Part model, mm, in its own coordinate system. Face numbers are marked on the shaded views. A direction names the side the tool comes from. Coordinates: 2 decimals unless noted, no trailing zeros. Loops run counter-clockwise (first coordinate to the right, second up) from the corner with the lowest first, then second, coordinate; pieces in that order, holes last. Notation, with made-up numbers: M 31,-8.5 L 72,-8.5 A20 cw 72,1.5 Z; hole C 7.5,58.5 d5. An arc over 180 degrees is marked long. Use a Markdown table: item, result. Add a question column.
1) Band-saw the part on C-C (z = -102.5). List the corners of the cut face in (x, y).
2) Tool access for the marked faces 1 and 2: list every direction of +Z, -Z, +X, -X, +Y, -Y with a clear straight run to the whole face (end or side of a thin tool).
3) Pin check, flat tips, straight feed: pin 1 Ø6 at (y, z) = (-45, -134.5) entering from +X; pin 2 Ø4 at (y, z) = (-28, -86) entering from -X; pin 3 Ø6 at (y, z) = (-46.5, -132.5) entering from -X. Stop position of each tip, or through.
4) Band-saw the part on B-B (y = 11). List the corners of the cut face in (x, z).
5) Band-saw the part on A-A (x = 0). List the corners of the cut face in (y, z).
6) Band-saw the part on D-D (y = -19). List the corners of the cut face in (x, z), plus the area to 3 significant figures.
7) Wall check: probe 1 along Y at (x, z) = (0, -138.5); probe 2 along X at (y, z) = (0, -142); probe 3 along Y at (x, z) = (0, -81). Give the ranges that are in metal, low to high. Write a range as from..to.
from build123d import *

# Parameters (mm, degrees)
SHELL1_T           = 3
SKETCH5_R          = 25
CUT_EXTRUDE3_DEPTH = 170.883652636
SKETCH6_W          = 64
SKETCH6_H          = 41
CUT_EXTRUDE4_DEPTH = 170.883652636


with BuildPart() as part:
    # Sketch2 → Revolve1 (revolve)
    with BuildSketch(Plane(origin=(0, 0, 0), x_dir=(0, 0, -1), z_dir=(1, 0, 0)), mode=Mode.PRIVATE) as revolve1_sk:
        with BuildLine():
            Line((76.080335522, 0), (147.580335522, 0))
            Line((147.580335522, 0), (147.580335522, 56.5))
            Line((147.580335522, 56.5), (132.580335522, 56.5))
            ThreePointArc((132.580335522, 56.5), (92.628802385, 39.951533137), (76.080335522, 0))
        make_face()
    revolve(revolve1_sk.sketch.rotate(Axis((0, 0, -76.080335522), (0, 0, 1)), 90), axis=Axis((0, 0, -76.080335522), (0, 0, 1)))

    # Shell1
    shell1_openings = [part.faces().sort_by_distance(p)[0] for p in [
        (0, 0, -147.580335522),
    ]]
    offset(amount=SHELL1_T, openings=shell1_openings, kind=Kind.INTERSECTION)

    # Sketch5 → Cut-Extrude3 (cut, through all)
    with BuildSketch(Plane.XY):
        with Locations(Location((0, 0, 0), (0, 0, 180))):
            Circle(SKETCH5_R)
    extrude(amount=-CUT_EXTRUDE3_DEPTH, mode=Mode.SUBTRACT)

    # Sketch6 → Cut-Extrude4 (cut, through all)
    with BuildSketch(Plane(origin=(0, 0, 0), x_dir=(1, 0, 0), z_dir=(0, 1, 0))):
        with Locations((0, 127.080335522)):
            Rectangle(SKETCH6_W, SKETCH6_H)
    extrude(amount=-CUT_EXTRUDE4_DEPTH, mode=Mode.SUBTRACT)


solid = part.part
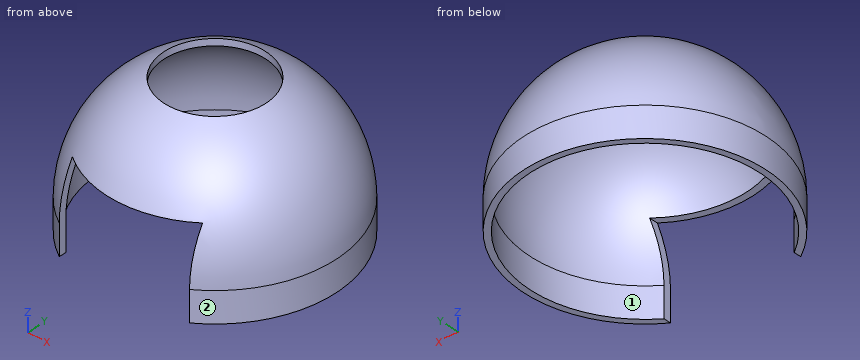
Entries:
| question | item | result |
|---|---|---|
| 1 | outline | C 0,0 d102.67; hole C 0,0 d95.65 |
| 2 | face 1 | -Z |
| 2 | face 2 | +Z, -Z |
| 3 | pin 1 | x = 42.15 |
| 3 | pin 2 | x = -28.28 |
| 3 | pin 3 | x = -40.6 |
| 4 | outline | M -58.47,-147.58 L -55.42,-147.58 L -55.42,-132.58 A55.42 cw -22.45,-81.91 L -22.45,-78.59 A58.47 ccw -58.47,-132.58 Z; M 22.45,-81.91 A55.42 cw 55.42,-132.58 L 55.42,-147.58 L 58.47,-147.58 L 58.47,-132.58 A58.47 ccw 22.45,-78.59 Z |
| 5 | outline | M -53.52,-106.58 L -50.16,-106.58 A56.5 cw -25,-81.91 L -25,-78.59 A59.5 ccw Z; M 25,-81.91 A56.5 cw 56.5,-132.58 L 56.5,-147.58 L 59.5,-147.58 L 59.5,-132.58 A59.5 ccw 25,-78.59 Z |
| 6 | outline | M -56.38,-147.58 L -53.21,-147.58 L -53.21,-132.58 A53.21 cw -16.25,-81.91 L -16.25,-78.59 A56.38 ccw -56.38,-132.58 Z; M 16.25,-81.91 A53.21 cw 53.21,-132.58 L 53.21,-147.58 L 56.38,-147.58 L 56.38,-132.58 A56.38 ccw 16.25,-78.59 Z |
| 6 | area | 537 mm2 |
| 7 | probe 1 | 56.5..59.5 |
| 7 | probe 2 | -59.5..-56.5, 56.5..59.5 |
| 7 | probe 3 | -29.66..-25, 25..29.66 |
